Input: part model. Units: mm. Frame: model coordinates. Round coordinates to 2 decimals unless told otherwise and drop trailing zeros. Order: outer loops, then holes, each group sorted by start corner. A loop starts at its lowest first (then second) coordinate and runs counter-clockwise, first axis right, second up. Notation, with made-up numbers: (42, 50.5) -> (55, 50.5) arc R25 ccw to (55, 63.5) -> close; hole circle Ø10 at (68.25, -37). An arc over 180 degrees is marked (long way). Use a Markdown table: item, result.
from build123d import *

# Parameters (mm, degrees)
SKETCH2_W          = 17.5
SKETCH2_H          = 440
CHAMFER1_SIZE      = 1.5
SKETCH3_R          = 0.5
CUT_EXTRUDE1_DEPTH = 3


with BuildPart() as part:
    # Sketch2 → Revolve1 (revolve)
    with BuildSketch(Plane.XY, mode=Mode.PRIVATE) as revolve1_sk:
        with Locations((8.75, 220)):
            Rectangle(SKETCH2_W, SKETCH2_H)
    revolve(revolve1_sk.sketch.rotate(Axis((0, 440, 0), (0, -1, 0)), 180), axis=Axis((0, 440, 0), (0, -1, 0)))

    # Chamfer1
    chamfer1_edges = [part.edges().sort_by_distance(p)[0] for p in [
        (17.5, 0, 0),
        (17.5, 440, 0),
    ]]
    chamfer(chamfer1_edges, length=CHAMFER1_SIZE)

    # Sketch3 → Cut-Extrude1 (cut)
    with BuildSketch(Plane.XZ):
        Circle(SKETCH3_R)
    extrude(amount=-CUT_EXTRUDE1_DEPTH, mode=Mode.SUBTRACT)


solid = part.part
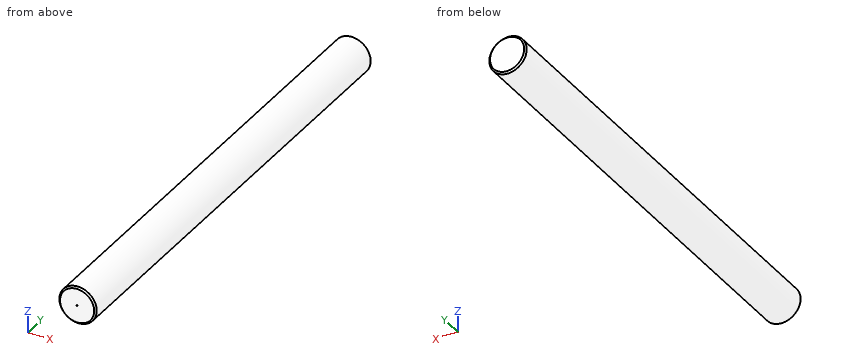
1) Ray query, probe 1 along Z at (x, y) = (0, 1.9); probe 2 along Z at (x, y) = (-0.5, 309.5); probe 3 along Z at (x, y) = (1.5, 251.5). Return the intervals inside material, ascending.
Answer key:
| item | result |
|---|---|
| probe 1 | z = -17.5 to -0.5, 0.5 to 17.5 |
| probe 2 | z = -17.49 to 17.49 |
| probe 3 | z = -17.44 to 17.44 |
2) Cut plane A-A on y = 145. Return loops of the section in (x, z).
Answer key:
| item | result |
|---|---|
| outline | circle Ø35 at (0, 0) |
3) Contact query for flat-ended pins moving along their axis: P1, Ø10, axis at x = 8.5, y = 377.5, coming from the +Z side; P2, Ø1, axis at y = 144, z = 9, coming from the -X side; P3, Ø6, axis at y = 148.5, z = -5, coming from the +X side. Output: stop coordinate, or through.
Answer key:
| item | result |
|---|---|
| P1 | stops at z = 17.15 |
| P2 | stops at x = -15.3 |
| P3 | stops at x = 17.39 |
